CAD build for the part. Positions are in the model's coordinates, mm. Round coordinates to 2 decimals unless told otherwise and drop trailing zeros. Write each loop counter-clockwise with the first axis right and the second up, starting at its lowest first coordinate (ties: lowest second). Pieces come first, ordered by that corner, then holes. Notation, with made-up numbers: (73, 15) - (90, 15) arc R22 cw to (90, 45) - close; hole circle Ø2 at (66, 80). An arc over 180 degrees is marked (long way). Put each result on its own line as item: value. Start each with the question number.
Item 1: Pin check, flat tip, straight feed: pin 1 Ø2.5 at (x, y) = (-55.25, -57.09) entering from -Z. Stop position of the tip, or through.
Item 2: Drill centre lines: line 1 (Y direction, x = 42.5, z = 1.3); line 2 (X direction, y = -38, z = 1.2); line 3 (X direction, y = 86.5, z = 0.55). Where is each one in solid material? Low to high. Write a range as from..to.
Item 3: Cut at A-A (z = 0.25). Give the cut face in (x, y).
```python
from build123d import *

# Parameters (mm, degrees)
SKETCH1_R           = 1.6
BOSS_EXTRUDE1_DEPTH = 1.5875
SKETCH3_W           = 12
SKETCH3_H           = 14
CUT_EXTRUDE1_DEPTH  = 125.589614038


with BuildPart() as part:
    # Sketch1 → Boss-Extrude1 (new body)
    with BuildSketch(Plane.XY):
        with BuildLine():
            Line((52.877308189, 101.03934739), (-47.122691811, 101.03934739))
            ThreePointArc((-47.122691811, 101.03934739), (-61.264827435, 95.181483014), (-67.122691811, 81.03934739))
            Line((-67.122691811, 81.03934739), (-67.122691811, -48.96065261))
            ThreePointArc((-67.122691811, -48.96065261), (-61.264827435, -63.102788233), (-47.122691811, -68.96065261))
            Line((-47.122691811, -68.96065261), (52.877308189, -68.96065261))
            ThreePointArc((52.877308189, -68.96065261), (67.019443812, -63.102788233), (72.877308189, -48.96065261))
            Line((72.877308189, -48.96065261), (72.877308189, 81.03934739))
            ThreePointArc((72.877308189, 81.03934739), (67.019443812, 95.181483014), (52.877308189, 101.03934739))
        make_face()
        with Locations((-55.254419795, -57.092380593)):
            Circle(SKETCH1_R, mode=Mode.SUBTRACT)
        with Locations((61.009036172, -57.092380593)):
            Circle(SKETCH1_R, mode=Mode.SUBTRACT)
        with Locations((61.009036172, 89.171075374)):
            Circle(SKETCH1_R, mode=Mode.SUBTRACT)
        with Locations((-55.254419795, 89.171075374)):
            Circle(SKETCH1_R, mode=Mode.SUBTRACT)
    extrude(amount=BOSS_EXTRUDE1_DEPTH)

    # Sketch3 → Cut-Extrude1 (cut, through all)
    with BuildSketch(Plane.XY.offset(1.5875)):
        with Locations((37.877308189, -43.96065261)):
            Rectangle(SKETCH3_W, SKETCH3_H)
    extrude(amount=-CUT_EXTRUDE1_DEPTH, mode=Mode.SUBTRACT)


solid = part.part
```
Output values:
1. pin 1: through
2. line 1: -68.96..-50.96, -36.96..101.04
2. line 2: -67.12..31.88, 43.88..72.88
2. line 3: -66.36..72.12
3. outline: (-67.12, -48.96) arc R20 ccw to (-47.12, -68.96) - (52.88, -68.96) arc R20 ccw to (72.88, -48.96) - (72.88, 81.04) arc R20 ccw to (52.88, 101.04) - (-47.12, 101.04) arc R20 ccw to (-67.12, 81.04) - close; hole circle Ø3.2 at (-55.25, -57.09); hole circle Ø3.2 at (-55.25, 89.17); hole (31.88, -50.96) - (43.88, -50.96) - (43.88, -36.96) - (31.88, -36.96) - close; hole circle Ø3.2 at (61.01, -57.09); hole circle Ø3.2 at (61.01, 89.17)
